from build123d import *

# Parameters (mm, degrees)
SKETCH1_W           = 20
SKETCH1_H           = 20
BOSS_EXTRUDE1_DEPTH = 7
SKETCH2_R           = 2.75
CUT_EXTRUDE1_DEPTH  = 8
BOSS_EXTRUDE2_DEPTH = 20
FILLET1_R           = 10


with BuildPart() as part:
    # Sketch1 → Boss-Extrude1 (new body)
    with BuildSketch(Plane.XY):
        with Locations((10, -10)):
            Rectangle(SKETCH1_W, SKETCH1_H)
    extrude(amount=BOSS_EXTRUDE1_DEPTH)

    # Sketch2 → Cut-Extrude1 (cut, through all)
    with BuildSketch(Plane.XY.offset(7)):
        with Locations((10, -10)):
            Circle(SKETCH2_R)
    extrude(amount=-CUT_EXTRUDE1_DEPTH, mode=Mode.SUBTRACT)

    # Sketch3 → Boss-Extrude2 (add)
    with BuildSketch(Plane(origin=(0, 0, 0), x_dir=(1, 0, 0), z_dir=(0, 1, 0))):
        Polygon((0, -7), (1.423068417, -31.959464663), (0.659996677, -35.607013498), (4.47015192, -36.404102701), (5.5, -31.481339917), (4.104191952, -7), align=None)
        Polygon((15.895808048, -7), (20, -7), (18.576931583, -31.959464663), (19.340003323, -35.607013498), (15.52984808, -36.404102701), (14.5, -31.481339917), align=None)
    extrude(amount=-BOSS_EXTRUDE2_DEPTH)

    # Fillet1
    fillet1_edges = [part.edges().sort_by_distance(p)[0] for p in [
        (5.5, -10, 31.481339917),
        (14.5, -10, 31.481339917),
    ]]
    fillet(fillet1_edges, radius=FILLET1_R)


solid = part.part
Geometry check sheet. Reference: the model listing, model coordinates, mm. A direction names the side the tool comes from. Coordinates: 2 decimals unless noted, no trailing zeros. Order: outer loops, then holes, each group sorted by start corner. A loop starts at its lowest first (then second) coordinate and runs counter-clockwise, first axis right, second up. Notation, with made-up numbers: (-17.5, 3) -> (6.5, 3) arc R30 ccw to (6.5, 35) -> close; hole circle Ø11 at (2.5, 20). An arc over 180 degrees is marked (long way). Use a Markdown table: item, result. Add a question column.
1. Cross-section at C-C (z = 22). Enter the section's corners in (x, y).
2. Cross-section at D-D (y = -2). Enter the section's corners in (x, z), and give its area (3 significant figures).
3. Set-up check for faces 1 (the face through (15.156, -9.86, 34.616)), 2 (the face through (1.047, -9.86, 33.758)), 3 (the face through (14.586, -10.14, 31.456)), 4 (the face through (18.953, -9.86, 33.758)), 5 (the face through (2.54, -9.86, 36)): record each of +Z, -Z, +X, -X, +Y, -Y from which the full face is reachable in a straight line by a thin tool's end or side.
4. Mould release check, pull along X, two halves, no side actions. Record for faces 6 (the face through (4.844, -9.86, 34.616)), 7 (the face through (0.7, -9.9, 19.3)), 8 (the face through (15.226, -9.86, 18.742)), 9 (the face through (19.3, -9.9, 19.3)): pulls with the +X half, pulls with the -X half, needs draft (parallel to the pull), parting line crosses it, or undercut.
5. Cross-section at A-A (y = -10). Enter the section's corners in (x, z).
6. Go/stop test with flat-tipped pins: pin 1 Ø5 at (y, z) = (-10.5, 10.5) entering from +X; pin 2 Ø6 at (y, z) = (-2.5, 25.5) entering from +X; pin 3 Ø7 at (x, y) = (10, -10) entering from +Z. Record where each tip stops, or that it passes through.
7. Material ranges on L1, parallel to Y at x = 10, z = 3.25; L2, parallel to Z at x = 12.25, y = -8.25; L3, parallel to X at y = -6.75, z = 23, recorded low to high.
8. Cross-section at B-B (x = 10). Enter the section's corners in (y, z), and give its area (4 significant figures).
Filled sheet:
| question | item | result |
|---|---|---|
| 1 | outline | (0.86, -20) -> (4.96, -20) -> (4.96, 0) -> (0.86, 0) -> close; (15.04, -20) -> (19.14, -20) -> (19.14, 0) -> (15.04, 0) -> close |
| 2 | outline | (0, 0) -> (20, 0) -> (20, 7) -> (18.58, 31.96) -> (19.34, 35.61) -> (15.53, 36.4) -> (14.77, 32.78) arc R10 ccw to (14.58, 30.16) -> (15.9, 7) -> (4.1, 7) -> (5.42, 30.16) arc R10 ccw to (5.23, 32.78) -> (4.47, 36.4) -> (0.66, 35.61) -> (1.42, 31.96) -> (0, 7) -> close |
| 2 | area | 377 mm2 |
| 3 | face 1 | +Z, +Y, -Y |
| 3 | face 2 | -X, +Y, -Y |
| 3 | face 3 | +Y, -Y |
| 3 | face 4 | +X, +Y, -Y |
| 3 | face 5 | +Z, -X, +Y, -Y |
| 4 | face 6 | undercut |
| 4 | face 7 | pulls with the -X half |
| 4 | face 8 | undercut |
| 4 | face 9 | pulls with the +X half |
| 5 | outline | (0, 0) -> (7.25, 0) -> (7.25, 7) -> (4.1, 7) -> (5.42, 30.16) arc R10 ccw to (5.23, 32.78) -> (4.47, 36.4) -> (0.66, 35.61) -> (1.42, 31.96) -> (0, 7) -> close; (12.75, 0) -> (20, 0) -> (20, 7) -> (18.58, 31.96) -> (19.34, 35.61) -> (15.53, 36.4) -> (14.77, 32.78) arc R10 ccw to (14.58, 30.16) -> (15.9, 7) -> (12.75, 7) -> close |
| 6 | pin 1 | x = 19.94 |
| 6 | pin 2 | x = 19.12 |
| 6 | pin 3 | z = 7 |
| 7 | L1 | -20 to -12.75, -7.25 to 0 |
| 7 | L2 | 0 to 7 |
| 7 | L3 | 0.91 to 5.02, 14.98 to 19.09 |
| 8 | outline | (-20, 0) -> (-12.75, 0) -> (-12.75, 7) -> (-20, 7) -> close; (-7.25, 0) -> (0, 0) -> (0, 7) -> (-7.25, 7) -> close |
| 8 | area | 101.5 mm2 |
